```python
from build123d import *

# Parameters (mm, degrees)
BOSS_EXTRUDE1_DEPTH       = 20
SKETCH2_W                 = 20
SKETCH2_H                 = 40
CUT_EXTRUDE1_DEPTH        = 142.509716981
SHELL1_T                  = -2
SHELL1_THICKNESS_2_FACE_W = 20
SHELL1_THICKNESS_2_FACE_H = 18
SHELL1_THICKNESS_2_DEPTH  = 3
SHELL1_THICKNESS_3_FACE_W = 18
SHELL1_THICKNESS_3_FACE_H = 20
SHELL1_THICKNESS_3_DEPTH  = 3
CUT_EXTRUDE14_REACH       = 110.167
SKETCH34_R                = 2.5
SKETCH3_W                 = 2.5
SKETCH3_H                 = 10
BOSS_EXTRUDE2_DEPTH       = 5
FILLET2_R                 = 5
CUT_EXTRUDE3_REACH        = 149.838
SKETCH6_R                 = 1.5
SKETCH21_R                = 2.5
SKETCH21_R_2              = 1.5
BOSS_EXTRUDE10_DEPTH      = 2.5
BOSS_EXTRUDE10_DRAFT      = 3
MIRROR7_COPY_1_SKETCH_R   = 2.5
MIRROR7_COPY_1_SKETCH_R_2 = 1.5
MIRROR7_COPY_1_DEPTH      = 2.5
MIRROR7_COPY_1_DRAFT      = 3
SKETCH26_W                = 5
SKETCH26_H                = 10
CUT_EXTRUDE8_DEPTH        = 2
SKETCH7_W                 = 2.5
SKETCH7_H                 = 10
BOSS_EXTRUDE4_DEPTH       = 5
FILLET4_R                 = 5
SKETCH22_R                = 2.5
BOSS_EXTRUDE11_DEPTH      = 2.5
BOSS_EXTRUDE11_TAPER      = 3
SKETCH23_R                = 1.5
CUT_EXTRUDE7_DEPTH        = 10
SKETCH27_W                = 5
SKETCH27_H                = 10
CUT_EXTRUDE9_DEPTH        = 2
SKETCH10_W                = 2.5
SKETCH10_H                = 10
BOSS_EXTRUDE6_DEPTH       = 5
FILLET6_R                 = 5
SKETCH28_R                = 2.5
BOSS_EXTRUDE12_DEPTH      = 2.5
BOSS_EXTRUDE12_TAPER      = 3
SKETCH29_R                = 1.5
CUT_EXTRUDE10_DEPTH       = 10
SKETCH30_W                = 5
SKETCH30_H                = 10
CUT_EXTRUDE11_DEPTH       = 2
SKETCH13_W                = 2.5
SKETCH13_H                = 10
BOSS_EXTRUDE8_DEPTH       = 5
FILLET8_R                 = 5
SKETCH31_R                = 2.5
BOSS_EXTRUDE13_DEPTH      = 2.5
BOSS_EXTRUDE13_TAPER      = 3
SKETCH32_R                = 1.5
CUT_EXTRUDE12_DEPTH       = 10
SKETCH33_W                = 5
SKETCH33_H                = 10
CUT_EXTRUDE13_DEPTH       = 2
SKETCH38_W                = 2
SKETCH38_H                = 30
BOSS_EXTRUDE14_DEPTH      = 15
BOSS_EXTRUDE15_DEPTH      = 5
CUT_EXTRUDE15_DEPTH       = 21
CUT_EXTRUDE15_DEPTH_BACK  = 1
SKETCH40_R                = 1.25


with BuildPart() as part:
    # Sketch1 → Boss-Extrude1 (new body)
    with BuildSketch(Plane.XY):
        Polygon((58, 114), (58, 115), (80, 115), (80, 20), (60, 0), (0, 0), (-10, 25), (-10, 105), (11, 105), (11, 110), (12, 110), (34, 110), (34, 115), (35, 115), (57, 115), (57, 114), align=None)
    extrude(amount=BOSS_EXTRUDE1_DEPTH)

    # Sketch2 → Cut-Extrude1 (cut, through all)
    with BuildSketch(Plane.XY.offset(20)):
        with Locations((70, 45)):
            Rectangle(SKETCH2_W, SKETCH2_H)
    extrude(amount=-CUT_EXTRUDE1_DEPTH, mode=Mode.SUBTRACT)

    # Shell1
    shell1_openings = [part.faces().sort_by_distance(p)[0] for p in [
        (32.550473836, 58.500730419, 20),
    ]]
    offset(amount=SHELL1_T, openings=shell1_openings, kind=Kind.INTERSECTION)

    # Shell1 thickness 2 face (on inner face of the shell) → Shell1 thickness 2 (add)
    with BuildSketch(Plane(origin=(68, 23, 11), x_dir=(1, 0, 0), z_dir=(0, 1, 0))):
        Rectangle(SHELL1_THICKNESS_2_FACE_W, SHELL1_THICKNESS_2_FACE_H)
    extrude(amount=-SHELL1_THICKNESS_2_DEPTH)

    # Shell1 thickness 3 face (on inner face of the shell) → Shell1 thickness 3 (add)
    with BuildSketch(Plane(origin=(68, 67, 11), x_dir=(0, 0, -1), z_dir=(0, -1, 0))):
        Rectangle(SHELL1_THICKNESS_3_FACE_W, SHELL1_THICKNESS_3_FACE_H)
    extrude(amount=-SHELL1_THICKNESS_3_DEPTH)

    # Cut-Extrude14: up to this face of the body (flat: up to its plane)
    cut_extrude14_end = Plane(part.part.faces().sort_by_distance((67.585786438, 20, 11))[0])
    # Sketch34 → Cut-Extrude14 (cut, up to the picked face)
    with BuildSketch(Plane(origin=(0, 70, 0), x_dir=(1, 0, 0), z_dir=(0, 1, 0)), mode=Mode.PRIVATE) as cut_extrude14_sk1:
        with Locations(Location((70, -11, 0), (0, 0, 270))):
            Circle(SKETCH34_R)
    cut_extrude14_tool1 = split(extrude(cut_extrude14_sk1.sketch, amount=-CUT_EXTRUDE14_REACH, mode=Mode.PRIVATE), bisect_by=cut_extrude14_end, keep=Keep.BOTH, mode=Mode.PRIVATE)
    add(cut_extrude14_tool1.solids().sort_by(Axis((70, 70, 11), (0, -1, 0)))[0], mode=Mode.SUBTRACT)

    # Sketch3 → Boss-Extrude2 (add)
    with BuildSketch(Plane(origin=(0, 115, 0), x_dir=(1, 0, 0), z_dir=(0, 1, 0))):
        with Locations((65.25, -13)):
            Rectangle(SKETCH3_W, SKETCH3_H)
        with Locations((72.75, -13)):
            Rectangle(SKETCH3_W, SKETCH3_H)
    extrude(amount=BOSS_EXTRUDE2_DEPTH)

    # Fillet2
    fillet2_edges = [part.edges().sort_by_distance(p)[0] for p in [
        (65.25, 120, 8),
        (65.25, 120, 18),
        (72.75, 120, 8),
        (72.75, 120, 18),
    ]]
    fillet(fillet2_edges, radius=FILLET2_R - 0.0001)  # a hair under: the kernel refuses the full size

    # Cut-Extrude3: up to this face of the body (flat: up to its plane)
    cut_extrude3_end = Plane(part.part.faces().sort_by_distance((64, 117.122079053, 13))[0])
    # Sketch6 → Cut-Extrude3 (cut, up to the picked face)
    with BuildSketch(Plane(origin=(74, 0, 0), x_dir=(0, 0, -1), z_dir=(1, 0, 0)), mode=Mode.PRIVATE) as cut_extrude3_sk1:
        with Locations((-13, 117.5)):
            Circle(SKETCH6_R)
    cut_extrude3_tool1 = split(extrude(cut_extrude3_sk1.sketch, amount=-CUT_EXTRUDE3_REACH, mode=Mode.PRIVATE), bisect_by=cut_extrude3_end, keep=Keep.BOTH, mode=Mode.PRIVATE)
    add(cut_extrude3_tool1.solids().sort_by(Axis((74, 117.5, 13), (-1, 0, 0)))[0], mode=Mode.SUBTRACT)


with BuildPart() as boss_extrude10_tool:
    # Sketch21 → Boss-Extrude10 (with draft: the straight prism first)
    with BuildSketch(Plane(origin=(66.5, 0, 0), x_dir=(0, 0, -1), z_dir=(1, 0, 0))):
        with Locations((-13, 117.5)):
            Circle(SKETCH21_R)
        with Locations((-13, 117.5)):
            Circle(SKETCH21_R_2, mode=Mode.SUBTRACT)
    extrude(amount=BOSS_EXTRUDE10_DEPTH)
    # Boss-Extrude10: the draft: its side faces are tilted about the plane it starts from
    boss_extrude10_sides = [boss_extrude10_tool.faces().sort_by_distance(p)[0] for p in [
        (67.75, 117.5, 15.5),
        (67.75, 117.5, 14.5),
    ]]
    draft(boss_extrude10_sides, Plane(origin=(66.5, 0, 0), x_dir=(0, 0, -1), z_dir=(1, 0, 0)), BOSS_EXTRUDE10_DRAFT)


with BuildPart() as part_1:
    add(part.part)

    # Boss-Extrude10: add boss_extrude10_tool
    add(boss_extrude10_tool.part)


with BuildPart() as mirror7_copy_1_tool:
    # Mirror7 copy 1 sketch → Mirror7 copy 1 (with draft: the straight prism first)
    with BuildSketch(Plane(origin=(71.5, 0, 0), x_dir=(0, 0, -1), z_dir=(-1, 0, 0))):
        with Locations((-13, -117.5)):
            Circle(MIRROR7_COPY_1_SKETCH_R)
        with Locations((-13, -117.5)):
            Circle(MIRROR7_COPY_1_SKETCH_R_2, mode=Mode.SUBTRACT)
    extrude(amount=MIRROR7_COPY_1_DEPTH)
    # Mirror7 copy 1: the draft: its side faces are tilted about the plane it starts from
    mirror7_copy_1_sides = [mirror7_copy_1_tool.faces().sort_by_distance(p)[0] for p in [
        (70.25, 117.5, 15.5),
        (70.25, 117.5, 14.5),
    ]]
    draft(mirror7_copy_1_sides, Plane(origin=(71.5, 0, 0), x_dir=(0, 0, -1), z_dir=(-1, 0, 0)), MIRROR7_COPY_1_DRAFT)


with BuildPart() as part_2:
    add(part_1.part)

    # Mirror7 copy 1: add mirror7_copy_1_tool
    add(mirror7_copy_1_tool.part)

    # Sketch26 → Cut-Extrude8 (cut)
    with BuildSketch(Plane(origin=(0, 115, 0), x_dir=(1, 0, 0), z_dir=(0, 1, 0))):
        with Locations((69, -13)):
            Rectangle(SKETCH26_W, SKETCH26_H)
    extrude(amount=-CUT_EXTRUDE8_DEPTH, mode=Mode.SUBTRACT)

    # Sketch7 → Boss-Extrude4 (add)
    with BuildSketch(Plane(origin=(0, 115, 0), x_dir=(1, 0, 0), z_dir=(0, 1, 0))):
        with Locations((41.25, -13)):
            Rectangle(SKETCH7_W, SKETCH7_H)
        with Locations((48.75, -13)):
            Rectangle(SKETCH7_W, SKETCH7_H)
    extrude(amount=BOSS_EXTRUDE4_DEPTH)

    # Fillet4
    fillet4_edges = [part_2.edges().sort_by_distance(p)[0] for p in [
        (41.25, 120, 8),
        (41.25, 120, 18),
        (48.75, 120, 8),
        (48.75, 120, 18),
    ]]
    fillet(fillet4_edges, radius=FILLET4_R - 0.0001)  # a hair under: the kernel refuses the full size

    # Sketch22 → Boss-Extrude11 (add)
    with BuildSketch(Plane(origin=(42.5, 0, 0), x_dir=(0, 0, -1), z_dir=(1, 0, 0))):
        with Locations((-13, 117.5)):
            Circle(SKETCH22_R)
    boss_extrude11 = extrude(amount=BOSS_EXTRUDE11_DEPTH, taper=BOSS_EXTRUDE11_TAPER)

    # Mirror8: Boss-Extrude11 across plane
    add(boss_extrude11.mirror(Plane(origin=(45, 117.5, 13), x_dir=(0, 0, 1), z_dir=(1, 0, 0))))

    # Sketch23 → Cut-Extrude7 (cut)
    with BuildSketch(Plane(origin=(50, 0, 0), x_dir=(0, 0, -1), z_dir=(1, 0, 0))):
        with Locations((-13, 117.5)):
            Circle(SKETCH23_R)
    extrude(amount=-CUT_EXTRUDE7_DEPTH, mode=Mode.SUBTRACT)

    # Sketch27 → Cut-Extrude9 (cut)
    with BuildSketch(Plane(origin=(0, 115, 0), x_dir=(1, 0, 0), z_dir=(0, 1, 0))):
        with Locations((45, -13)):
            Rectangle(SKETCH27_W, SKETCH27_H)
    extrude(amount=-CUT_EXTRUDE9_DEPTH, mode=Mode.SUBTRACT)

    # Sketch10 → Boss-Extrude6 (add)
    with BuildSketch(Plane(origin=(0, 110, 0), x_dir=(1, 0, 0), z_dir=(0, 1, 0))):
        with Locations((19.25, -13)):
            Rectangle(SKETCH10_W, SKETCH10_H)
        with Locations((26.75, -13)):
            Rectangle(SKETCH10_W, SKETCH10_H)
    extrude(amount=BOSS_EXTRUDE6_DEPTH)

    # Fillet6
    fillet6_edges = [part_2.edges().sort_by_distance(p)[0] for p in [
        (19.25, 115, 18),
        (19.25, 115, 8),
        (26.75, 115, 8),
        (26.75, 115, 18),
    ]]
    fillet(fillet6_edges, radius=FILLET6_R - 0.0001)  # a hair under: the kernel refuses the full size

    # Sketch28 → Boss-Extrude12 (add)
    with BuildSketch(Plane(origin=(20.5, 0, 0), x_dir=(0, 0, -1), z_dir=(1, 0, 0))):
        with Locations((-13, 112.5)):
            Circle(SKETCH28_R)
    boss_extrude12 = extrude(amount=BOSS_EXTRUDE12_DEPTH, taper=BOSS_EXTRUDE12_TAPER)

    # Mirror9: Boss-Extrude12 across plane
    add(boss_extrude12.mirror(Plane(origin=(23, 112.5, 13), x_dir=(0, 0, 1), z_dir=(1, 0, 0))))

    # Sketch29 → Cut-Extrude10 (cut)
    with BuildSketch(Plane(origin=(28, 0, 0), x_dir=(0, 0, -1), z_dir=(1, 0, 0))):
        with Locations((-13, 112.5)):
            Circle(SKETCH29_R)
    extrude(amount=-CUT_EXTRUDE10_DEPTH, mode=Mode.SUBTRACT)

    # Sketch30 → Cut-Extrude11 (cut)
    with BuildSketch(Plane(origin=(0, 110, 0), x_dir=(1, 0, 0), z_dir=(0, 1, 0))):
        with Locations((23, -13)):
            Rectangle(SKETCH30_W, SKETCH30_H)
    extrude(amount=-CUT_EXTRUDE11_DEPTH, mode=Mode.SUBTRACT)

    # Sketch13 → Boss-Extrude8 (add)
    with BuildSketch(Plane(origin=(0, 105, 0), x_dir=(1, 0, 0), z_dir=(0, 1, 0))):
        with Locations((-2.75, -13)):
            Rectangle(SKETCH13_W, SKETCH13_H)
        with Locations((4.75, -13)):
            Rectangle(SKETCH13_W, SKETCH13_H)
    extrude(amount=BOSS_EXTRUDE8_DEPTH)

    # Fillet8
    fillet8_edges = [part_2.edges().sort_by_distance(p)[0] for p in [
        (-2.75, 110, 18),
        (-2.75, 110, 8),
        (4.75, 110, 8),
        (4.75, 110, 18),
    ]]
    fillet(fillet8_edges, radius=FILLET8_R - 0.0001)  # a hair under: the kernel refuses the full size

    # Sketch31 → Boss-Extrude13 (add)
    with BuildSketch(Plane(origin=(-1.5, 0, 0), x_dir=(0, 0, -1), z_dir=(1, 0, 0))):
        with Locations((-13, 107.5)):
            Circle(SKETCH31_R)
    boss_extrude13 = extrude(amount=BOSS_EXTRUDE13_DEPTH, taper=BOSS_EXTRUDE13_TAPER)

    # Mirror10: Boss-Extrude13 across plane
    add(boss_extrude13.mirror(Plane(origin=(1, 107.5, 13), x_dir=(0, 0, 1), z_dir=(1, 0, 0))))

    # Sketch32 → Cut-Extrude12 (cut)
    with BuildSketch(Plane(origin=(6, 0, 0), x_dir=(0, 0, -1), z_dir=(1, 0, 0))):
        with Locations((-13, 107.5)):
            Circle(SKETCH32_R)
    extrude(amount=-CUT_EXTRUDE12_DEPTH, mode=Mode.SUBTRACT)

    # Sketch33 → Cut-Extrude13 (cut)
    with BuildSketch(Plane(origin=(0, 105, 0), x_dir=(1, 0, 0), z_dir=(0, 1, 0))):
        with Locations((1, -13)):
            Rectangle(SKETCH33_W, SKETCH33_H)
    extrude(amount=-CUT_EXTRUDE13_DEPTH, mode=Mode.SUBTRACT)

    # Sketch38 → Boss-Extrude14 (add)
    with BuildSketch(Plane.XY.offset(2)):
        with Locations((56, 97)):
            Rectangle(SKETCH38_W, SKETCH38_H)
    extrude(amount=BOSS_EXTRUDE14_DEPTH)

    # Sketch39 → Boss-Extrude15 (add)
    with BuildSketch(Plane.XY.offset(2)):
        Polygon((66, 98.2), (66, 100.2), (71, 100.2), (71, 90.2), (69, 90.2), (69, 98.2), align=None)
    extrude(amount=BOSS_EXTRUDE15_DEPTH)

    # Sketch40 → Cut-Extrude15 (cut, two sides: drawn at the far end of the back side and taken through both)
    with BuildSketch(Plane(origin=(57, 0, 0), x_dir=(0, 0, -1), z_dir=(1, 0, 0)).offset(-CUT_EXTRUDE15_DEPTH_BACK)):
        with Locations(Location((-13.5, 105, 0), (0, 0, 180))):
            Circle(SKETCH40_R)
    extrude(amount=CUT_EXTRUDE15_DEPTH + CUT_EXTRUDE15_DEPTH_BACK, mode=Mode.SUBTRACT)


solid = part_2.part
```
Input: part model. Units: mm. Frame: model coordinates. A direction names the side the tool comes from. Round coordinates to 2 decimals unless told otherwise and drop trailing zeros. Order: outer loops, then holes, each group sorted by start corner. A loop starts at its lowest first (then second) coordinate and runs counter-clockwise, first axis right, second up. Notation, with made-up numbers: (55.5, -8.5) - (69.5, -8.5) arc R23 ccw to (69.5, 17.5) - close; hole circle Ø4 at (49, 55). An arc over 180 degrees is marked (long way). One line per question, with ' | ' between items. Start each with the question number.
1) Ray query, probe 1 along Y at (x, z) = (56.45, 13.5); probe 2 along X at (y, z) = (106.5, 2.5); probe 3 along X at (y, z) = (69, 14.75). Return the intervals inside material, ascending.
2) Cut plane A-A, the plane z = 5.25. Give the number of separate pieces and of enclosed holes in the cut face, then the cut area to 3 significant figures.
3) Cut plane B-B, the plane x = 15.5. Return the cut outline in (y, z), then the cut area to 3 significant figures.
4) Contact query for flat-ended pins moving along their axis: P1, Ø6, axis at x = 12, y = 46, coming from the +Z side; P2, Ø1.5, axis at x = 53, z = 5, coming from the -Y side; P3, Ø5.5, axis at x = 68, z = 4.5, coming from the +Y side; P4, Ø6, axis at x = 67, z = 11, coming from the -Y side. Output: stop coordinate, or through.
5) Set-up query: faces 4 (the flat face through (48, 113, 11)), 5 (the flat face through (6, 105.8, 13.1)), 6 (the cylindrical face through (-3, 108, 17)), 7 (the cylindrical face through (27, 113, 9)). Return all of +Z, -Z, +X, -X, +Y, -Y with unobstructed straight access to the full face (end or side cutting, diameter ignored); none if empty.
6) Cut plane D-D, the plane x = 62.5. Return the cut outline in (y, z), then the cut area to 3 significant figures.
7) Pull-direction query (Z, two-part tool) for faces 1 (the cylindrical face through (73, 118, 17)), 2 (the flat face through (40, 115.8, 13.1)), 3 (the flat face through (25.5, 110, 12)); classes: +Z half, -Z half, draft (parallel to the pull), parting line (faces both ways), or undercut.
8) Cut plane C-C, the plane y = 74.5. Return the cut outline in (x, z).
Worked out:
1) probe 1: y = 0 to 2, 82 to 103.75, 106.25 to 115 | probe 2: x = 11 to 13, 55 to 57, 78 to 80 | probe 3: x = -10 to -8, 58 to 80
2) separate pieces: 2 | enclosed holes: 1 | area: 1,060 mm^2
3) outline: (0, 0) - (110, 0) - (110, 20) - (108, 20) - (108, 2) - (2, 2) - (2, 20) - (0, 20) - close | area: 292 mm^2
4) P1: stops at z = 2 | P2: stops at y = 0 | P3: stops at y = 115 | P4: stops at y = 4
5) face 4: +Z | face 5: +Z, -Z, +Y | face 6: +Z, -X, +Y | face 7: -Z, -X, +Y
6) outline: (2.5, 0) - (25, 0) - (25, 20) - (20, 20) - (20, 2) - (5.33, 2) - (5.33, 20) - (2.5, 20) - close; (65, 0) - (115, 0) - (115, 20) - (113, 20) - (113, 2) - (70, 2) - (70, 20) - (65, 20) - close | area: 412 mm^2
7) face 1: +Z half | face 2: draft | face 3: undercut
8) outline: (-10, 0) - (80, 0) - (80, 20) - (78, 20) - (78, 2) - (-8, 2) - (-8, 20) - (-10, 20) - close
